Verification items for the finished model (mm, model axes). Give positions to 0.01 mm unless a question says otherwise; leave off trailing zeros. Answer as CSV lines item,"result".
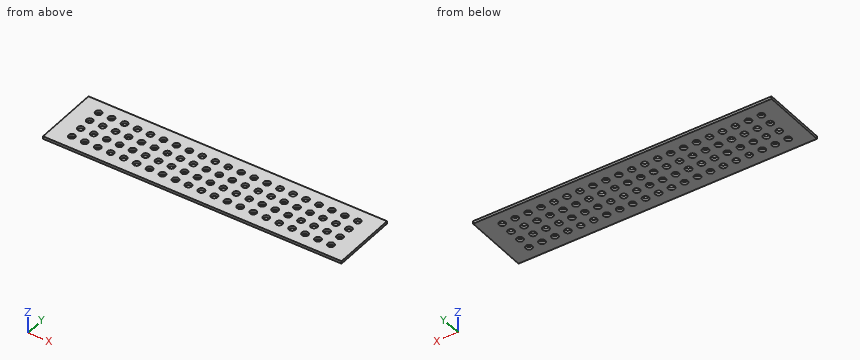
```python
from build123d import *

# Parameters (mm, degrees)
BOX_W        = 115
BOX_H        = 25.4
BOX_DEPTH    = 1
SKETCH_R     = 1.25
POCKET_DEPTH = 5


with BuildPart() as part:
    # Box → Box (new body)
    with BuildSketch(Plane.XY):
        with Locations((57.5, 12.7)):
            Rectangle(BOX_W, BOX_H)
    extrude(amount=BOX_DEPTH)

    # Sketch (on Face6 of BaseFeature) → Pocket (cut)
    with BuildSketch(Plane.XY.offset(1)):
        with Locations((7.536244, 20.148321)):
            Circle(SKETCH_R)
        with Locations((12.526654, 20.150693)):
            Circle(SKETCH_R)
        with Locations((17.517064, 20.153065)):
            Circle(SKETCH_R)
        with Locations((22.507474, 20.155437)):
            Circle(SKETCH_R)
        with Locations((27.497884, 20.157809)):
            Circle(SKETCH_R)
        with Locations((32.488294, 20.160181)):
            Circle(SKETCH_R)
        with Locations((37.478704, 20.162553)):
            Circle(SKETCH_R)
        with Locations((42.469114, 20.164925)):
            Circle(SKETCH_R)
        with Locations((47.459524, 20.167297)):
            Circle(SKETCH_R)
        with Locations((52.449934, 20.169669)):
            Circle(SKETCH_R)
        with Locations((57.440344, 20.172041)):
            Circle(SKETCH_R)
        with Locations((62.430754, 20.174413)):
            Circle(SKETCH_R)
        with Locations((67.421164, 20.176785)):
            Circle(SKETCH_R)
        with Locations((72.411574, 20.179157)):
            Circle(SKETCH_R)
        with Locations((77.401984, 20.181529)):
            Circle(SKETCH_R)
        with Locations((82.392394, 20.183901)):
            Circle(SKETCH_R)
        with Locations((87.382804, 20.186273)):
            Circle(SKETCH_R)
        with Locations((92.373214, 20.188645)):
            Circle(SKETCH_R)
        with Locations((97.363624, 20.191017)):
            Circle(SKETCH_R)
        with Locations((102.354034, 20.193389)):
            Circle(SKETCH_R)
        with Locations((107.344444, 20.195761)):
            Circle(SKETCH_R)
        with Locations((7.538616, 15.157911)):
            Circle(SKETCH_R)
        with Locations((12.529026, 15.160283)):
            Circle(SKETCH_R)
        with Locations((17.519436, 15.162655)):
            Circle(SKETCH_R)
        with Locations((22.509846, 15.165027)):
            Circle(SKETCH_R)
        with Locations((27.500256, 15.167399)):
            Circle(SKETCH_R)
        with Locations((32.490666, 15.169771)):
            Circle(SKETCH_R)
        with Locations((37.481076, 15.172143)):
            Circle(SKETCH_R)
        with Locations((42.471486, 15.174515)):
            Circle(SKETCH_R)
        with Locations((47.461896, 15.176887)):
            Circle(SKETCH_R)
        with Locations((52.452306, 15.179259)):
            Circle(SKETCH_R)
        with Locations((57.442716, 15.181631)):
            Circle(SKETCH_R)
        with Locations((62.433126, 15.184003)):
            Circle(SKETCH_R)
        with Locations((67.423536, 15.186375)):
            Circle(SKETCH_R)
        with Locations((72.413946, 15.188747)):
            Circle(SKETCH_R)
        with Locations((77.404356, 15.191119)):
            Circle(SKETCH_R)
        with Locations((82.394766, 15.193491)):
            Circle(SKETCH_R)
        with Locations((87.385176, 15.195863)):
            Circle(SKETCH_R)
        with Locations((92.375586, 15.198235)):
            Circle(SKETCH_R)
        with Locations((97.365996, 15.200607)):
            Circle(SKETCH_R)
        with Locations((102.356406, 15.202979)):
            Circle(SKETCH_R)
        with Locations((107.346816, 15.205351)):
            Circle(SKETCH_R)
        with Locations((7.540988, 10.167501)):
            Circle(SKETCH_R)
        with Locations((12.531398, 10.169873)):
            Circle(SKETCH_R)
        with Locations((17.521808, 10.172245)):
            Circle(SKETCH_R)
        with Locations((22.512218, 10.174617)):
            Circle(SKETCH_R)
        with Locations((27.502628, 10.176989)):
            Circle(SKETCH_R)
        with Locations((32.493038, 10.179361)):
            Circle(SKETCH_R)
        with Locations((37.483448, 10.181733)):
            Circle(SKETCH_R)
        with Locations((42.473858, 10.184105)):
            Circle(SKETCH_R)
        with Locations((47.464268, 10.186477)):
            Circle(SKETCH_R)
        with Locations((52.454678, 10.188849)):
            Circle(SKETCH_R)
        with Locations((57.445088, 10.191221)):
            Circle(SKETCH_R)
        with Locations((62.435498, 10.193593)):
            Circle(SKETCH_R)
        with Locations((67.425908, 10.195965)):
            Circle(SKETCH_R)
        with Locations((72.416318, 10.198337)):
            Circle(SKETCH_R)
        with Locations((77.406728, 10.200709)):
            Circle(SKETCH_R)
        with Locations((82.397138, 10.203081)):
            Circle(SKETCH_R)
        with Locations((87.387548, 10.205453)):
            Circle(SKETCH_R)
        with Locations((92.377958, 10.207825)):
            Circle(SKETCH_R)
        with Locations((97.368368, 10.210197)):
            Circle(SKETCH_R)
        with Locations((102.358778, 10.212569)):
            Circle(SKETCH_R)
        with Locations((107.349188, 10.214941)):
            Circle(SKETCH_R)
        with Locations((7.54336, 5.177091)):
            Circle(SKETCH_R)
        with Locations((12.53377, 5.179463)):
            Circle(SKETCH_R)
        with Locations((17.52418, 5.181835)):
            Circle(SKETCH_R)
        with Locations((22.51459, 5.184207)):
            Circle(SKETCH_R)
        with Locations((27.505, 5.186579)):
            Circle(SKETCH_R)
        with Locations((32.49541, 5.188951)):
            Circle(SKETCH_R)
        with Locations((37.48582, 5.191323)):
            Circle(SKETCH_R)
        with Locations((42.47623, 5.193695)):
            Circle(SKETCH_R)
        with Locations((47.46664, 5.196067)):
            Circle(SKETCH_R)
        with Locations((52.45705, 5.198439)):
            Circle(SKETCH_R)
        with Locations((57.44746, 5.200811)):
            Circle(SKETCH_R)
        with Locations((62.43787, 5.203183)):
            Circle(SKETCH_R)
        with Locations((67.42828, 5.205555)):
            Circle(SKETCH_R)
        with Locations((72.41869, 5.207927)):
            Circle(SKETCH_R)
        with Locations((77.4091, 5.210299)):
            Circle(SKETCH_R)
        with Locations((82.39951, 5.212671)):
            Circle(SKETCH_R)
        with Locations((87.38992, 5.215043)):
            Circle(SKETCH_R)
        with Locations((92.38033, 5.217415)):
            Circle(SKETCH_R)
        with Locations((97.37074, 5.219787)):
            Circle(SKETCH_R)
        with Locations((102.36115, 5.222159)):
            Circle(SKETCH_R)
        with Locations((107.35156, 5.224531)):
            Circle(SKETCH_R)
    extrude(amount=-POCKET_DEPTH, mode=Mode.SUBTRACT)


solid = part.part
```
1) Section check A-A (z = 0.65). State how many separate pieces and enclosed holes the cut face has, and give its area (3 significant figures).
Reported:
separate pieces,"1"
enclosed holes,"84"
area,"2,510 mm²"
2) Scan lines: line 1 along Y through (x, z) = (51.5, 0.2); line 2 along Y through (x, z) = (68, 0.65). Record each from-to range of solid material in increasing order.
Reported:
line 1,"0 to 4.39, 6 to 9.38, 11 to 14.37, 15.99 to 19.36, 20.98 to 25.4"
line 2,"0 to 4.09, 6.32 to 9.09, 11.31 to 14.08, 16.3 to 19.07, 21.28 to 25.4"
3) Depth check by flat-ended pin: pin 1 (1.5 mm diameter, centred on x = 107.35, y = 15.21, fed in from -Z) (1 decimal). Enter the tip coordinate at first touch or a pass-through.
Reported:
pin 1,"through"
